from build123d import *

# Parameters (mm, degrees)
F0_R     = 4.064
F0_R_2   = 1.5875
F1_DEPTH = 3.175


with BuildPart() as f1:
    # F0 (on Top) → F1 (new body)
    with BuildSketch(Plane.XY):
        with BuildLine():
            ThreePointArc((-10.409411, 38.146532), (-19.071367, 31.560942), (-27.622774, 38.289456))
            ThreePointArc((-27.622774, 38.289456), (-33.321705, 43.939553), (-38.826343, 38.1))
            Line((-38.826343, 38.1), (-27.879121, 6.072861))
            ThreePointArc((-27.879121, 6.072861), (-18.693227, -0.445875), (-9.600745, 6.202533))
            ThreePointArc((-9.600745, 6.202533), (-9.600626, 6.2029), (-9.600506, 6.203266))
            Line((-9.600506, 6.203266), (0.799111, 38.1))
            ThreePointArc((0.799111, 38.1), (-4.781981, 43.704309), (-10.409411, 38.146532))
        make_face()
        with Locations((-18.761582, 9.189334)):
            Circle(F0_R, mode=Mode.SUBTRACT)
        with Locations((-33.226947, 38.335988)):
            Circle(F0_R_2, mode=Mode.SUBTRACT)
        with Locations((-4.805247, 38.1)):
            Circle(F0_R_2, mode=Mode.SUBTRACT)
    extrude(amount=F1_DEPTH)


solid = f1.part
Could you check a few things on this model? Use its own coordinates, in mm. Coordinates: 2 decimals unless noted, no trailing zeros. Write each loop counter-clockwise with the first axis right and the second up, starting at its lowest first coordinate (ties: lowest second). Pieces come first, ordered by that corner, then holes. Notation, with made-up numbers: (75.25, 50.5) - (84.25, 50.5) arc R30 ccw to (84.25, 80.5) - close; hole circle Ø11 at (63.5, 79). An arc over 180 degrees is marked (long way). Write item = value, one per line.
1) Please list where these lines run through material, in increasing order: line 1 (Y direction, x = -19, z = 0.3); line 2 (X direction, y = 38, z = 2.55); line 3 (X direction, y = 42, z = 2.8). Write a range as [from, to].
Result set:
line_1 = [-0.44, 5.13], [13.25, 31.56]
line_2 = [-38.79, -34.78], [-31.68, -27.54], [-10.45, -6.39], [-3.22, 0.77]
line_3 = [-37.47, -28.99], [-8.83, -0.78]
2) Will these pins go through, and if not, where does the flat tip stop? pin 1 Ø1 at (x, z) = (-15, 1) entering from -Y; pin 2 Ø1.5 at (y, z) = (28.5, 2) entering from -X; pin 3 Ø5 at (x, y) = (-30, 13.5) entering from -Z.
Result set:
pin_1 = 0.12
pin_2 = -35.8
pin_3 = 0
3) Suppose I cut it at D-D on y = 3.5. Please give me the cut outline in (x, z) (3 decimals), plus the area to 3 significant figures.
Result set:
outline = (-26.538, 0) - (-10.985, 0) - (-10.985, 3.175) - (-26.538, 3.175) - close
area = 49.4 mm2
4) We'd pull the mould along X, two halves only. Please class faces 1 (the cylindrical face through (-21.757, 11.936, 1.565)), 2 (the flat face through (-4.473, 21.928, 1.565)), 3 (the cylindrical face through (-3.952, 39.439, 1.565)), 4 (the flat face through (-19, 22, 3.175)): +X half, -X half, draft (parallel to the pull), parting line (faces both ways), or undercut.
Result set:
face_1 = undercut
face_2 = +X half
face_3 = undercut
face_4 = draft
5) Suppose I cut it at C-C on x = -31. Please give me the cut outline in (y, z) (3 decimals).
Result set:
outline = (15.203, 0) - (43.479, 0) - (43.479, 3.175) - (15.203, 3.175) - close
6) Suppose I cut it at B-B on z = 1.95. State how many separate pieces and enclosed holes the cut face has, plus the area to 3 significant figures.
Result set:
separate_pieces = 1
enclosed_holes = 3
area = 964 mm2
7) Suppose I cut it at A-A on y = 36. Please give me the cut outline in (x, z) (3 decimals), plus the area to 3 significant figures.
Result set:
outline = (-38.109, 0) - (-26.695, 0) - (-26.695, 3.175) - (-38.109, 3.175) - close; (-11.3, 0) - (0.114, 0) - (0.114, 3.175) - (-11.3, 3.175) - close
area = 72.5 mm2
